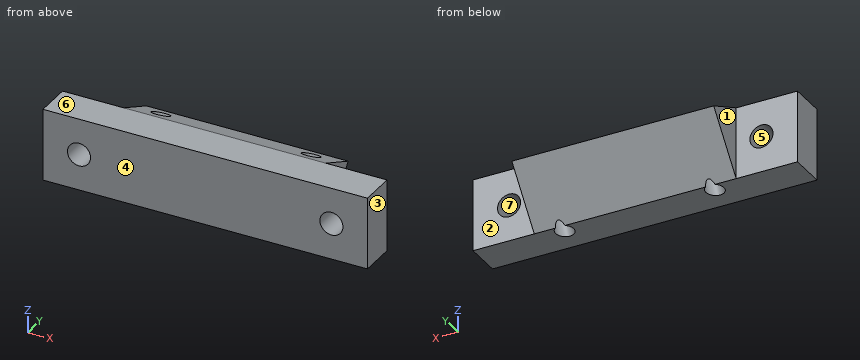
from build123d import *

# Parameters (mm, degrees)
SKETCH1_W           = 45
SKETCH1_H           = 10
SKETCH1_R           = 1.6
BOSS_EXTRUDE2_DEPTH = 5
BOSS_EXTRUDE3_DEPTH = 14
SKETCH4_R           = 1.25
CUT_EXTRUDE1_DEPTH  = 28


with BuildPart() as part:
    # Sketch1 → Boss-Extrude2 (new body)
    with BuildSketch(Plane(origin=(0, 0, 0), x_dir=(1, 0, 0), z_dir=(0, 1, 0))):
        Rectangle(SKETCH1_W, SKETCH1_H)
        with Locations((-17.5, 0)):
            Circle(SKETCH1_R, mode=Mode.SUBTRACT)
        with Locations((17.5, 0)):
            Circle(SKETCH1_R, mode=Mode.SUBTRACT)
    extrude(amount=BOSS_EXTRUDE2_DEPTH)

    # Sketch3 → Boss-Extrude3 (add, symmetric)
    with BuildSketch(Plane(origin=(0, 0, 0), x_dir=(0, 0, -1), z_dir=(1, 0, 0))):
        Polygon((-5, 5), (5, 5), (-2.316374038, 10.755054448), align=None)
    extrude(amount=BOSS_EXTRUDE3_DEPTH, both=True)

    # Sketch4 → Cut-Extrude1 (cut)
    with BuildSketch(Plane(origin=(0, 2.808142084, 6.022080132), x_dir=(1, 0, 0), z_dir=(0, 0.422618262, 0.906307787))):
        with Locations((-10.414, 5.593447626)):
            Circle(SKETCH4_R)
        with Locations((10.414, 5.593447626)):
            Circle(SKETCH4_R)
    extrude(amount=-CUT_EXTRUDE1_DEPTH, mode=Mode.SUBTRACT)


solid = part.part
Here's how the part is built. I have some questions about the finished solid (model axes, mm). Face numbers are marked on the shaded views. A direction names the side the tool comes from. Round coordinates to 2 decimals unless told otherwise and drop trailing zeros. Write each loop counter-clockwise with the first axis right and the second up, starting at its lowest first coordinate (ties: lowest second). Pieces come first, ordered by that corner, then holes. Notation, with made-up numbers: (20, 86) -> (71, 86) arc R22 ccw to (71, 122) -> close; hole circle Ø3 at (-24, -33.5). An arc over 180 degrees is marked (long way). One line per item, written item: value.
1) Suppose I cut it at D-D on x = 12.5. List the corners of the cut face in (y, z) for me.
Filled sheet:
outline: (0, -5) -> (5, -5) -> (10.76, 2.32) -> (5, 5) -> (0, 5) -> close
2) We'd pull the mould along Z, two halves only. Please class the marked faces 4, 5, 6 and 7: released by +Z, released by -Z, zero draft, split by the parting line, or undercut.
Filled sheet:
face 4: zero draft
face 5: undercut
face 6: released by +Z
face 7: undercut
3) I'm going to push flat-ended pins straight in: pin 1 Ø3 at (x, z) = (2.5, 4) entering from +Y; pin 2 Ø1.5 at (y, z) = (6.5, -1.5) entering from -X; pin 3 Ø5 at (x, z) = (14.5, -1) entering from +Y. Where does each tip first touch, or does it pass through?
Filled sheet:
pin 1: stops at y = 10.36
pin 2: stops at x = -14
pin 3: stops at y = 10.07
4) For the marked faces 1, 2 and 3, which set-ups out of +Z, -Z, +X, -X, +Y, -Y let a thin tool reach every point of the face, with its end or its side?
Filled sheet:
face 1: +Z, -Z, -X, +Y
face 2: +Z, -Z, +X, +Y
face 3: +Z, -Z, +X, +Y, -Y
5) If I drill on line 1 (X direction, y = 1.4, z = 0); line 2 (Z direction, x = -17.5, y = 3.55); line 3 (Y direction, x = 18.5, z = -4.5), over which ranges is the centre line in solid material (lowest first)? Write a range as [from, to].
Filled sheet:
line 1: x = [-22.5, -19.1], [-15.9, 15.9], [19.1, 22.5]
line 2: z = [-5, -1.6], [1.6, 5]
line 3: y = [0, 5]
6) Suppose I cut it at C-C on z = -0.75. Give the number of separate pieces and of enclosed holes in the cut face, plus the area to 3 significant figures.
Filled sheet:
separate pieces: 3
enclosed holes: 2
area: 280 mm2
7) Suppose I cut it at A-A on x = 17.5. List the corners of the cut face in (y, z) for me, plus the area to 3 significant figures.
Filled sheet:
outline: (0, -5) -> (5, -5) -> (5, -1.6) -> (0, -1.6) -> close; (0, 1.6) -> (5, 1.6) -> (5, 5) -> (0, 5) -> close
area: 34.0 mm2
8) Suppose I cut it at B-B on x = -18.5. List the corners of the cut face in (y, z) for me, plus the area to 3 significant figures.
Filled sheet:
outline: (0, -5) -> (5, -5) -> (5, -1.25) -> (0, -1.25) -> close; (0, 1.25) -> (5, 1.25) -> (5, 5) -> (0, 5) -> close
area: 37.5 mm2
